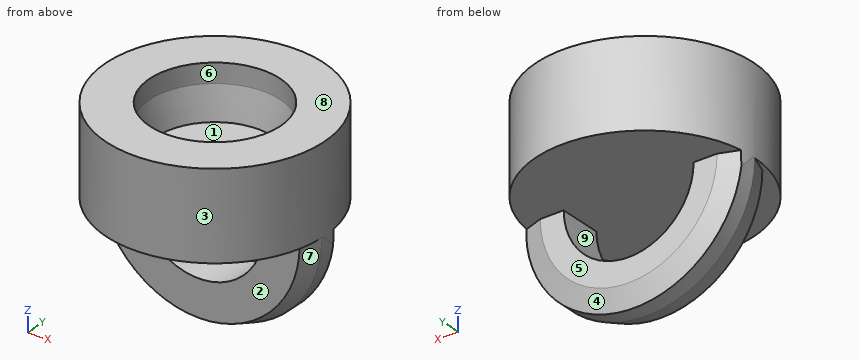
from build123d import *

# Parameters (mm, degrees)
SKETCH1_R                = 7.5
BOSS_EXTRUDE1_DEPTH      = 6
SKETCH2_R                = 4.5
CUT_EXTRUDE1_DEPTH       = 3.5
CHAMFER1_SIZE            = 0.5
CHAMFER1_SIZE2           = 2.165737937
BOSS_EXTRUDE2_DEPTH      = 1.5
BOSS_EXTRUDE2_DEPTH_BACK = 1.5
SKETCH4_OUTSIDE_W        = 22.028
SKETCH4_OUTSIDE_H        = 22.028
SKETCH4_OUTSIDE_R        = 7.5
CUT_EXTRUDE2_DEPTH       = 13.990381057
CHAMFER3_SIZE            = 1.37373871
CHAMFER3_SIZE_2          = 0.5


with BuildPart() as part:
    # Sketch1 → Boss-Extrude1 (new body)
    with BuildSketch(Plane.XY):
        Circle(SKETCH1_R)
    extrude(amount=BOSS_EXTRUDE1_DEPTH)

    # Sketch2 → Cut-Extrude1 (cut)
    with BuildSketch(Plane.XY.offset(6)):
        Circle(SKETCH2_R)
    extrude(amount=-CUT_EXTRUDE1_DEPTH, mode=Mode.SUBTRACT)

    # Chamfer1
    chamfer1_edges = [part.edges().sort_by_distance(p)[0] for p in [
        (-4.5, 0, 2.5),
    ]]
    chamfer1_side = [part.faces().sort_by_distance(p)[0] for p in [
        (0, 0, 2.5),
    ]]
    chamfer(chamfer1_edges, length=CHAMFER1_SIZE, length2=CHAMFER1_SIZE2, reference=chamfer1_side[0])

    # Sketch3 → Boss-Extrude2 (add, two sides: drawn at the far end of the back side and taken through both)
    with BuildSketch(Plane(origin=(0, 0, 0), x_dir=(1, 0, 0), z_dir=(0, 1, 0)).offset(-BOSS_EXTRUDE2_DEPTH_BACK)):
        with BuildLine():
            Line((-7.5, 0), (-4.5, 0))
            ThreePointArc((-4.5, 0), (0, 4.5), (4.5, 0))
            Line((4.5, 0), (7.5, 0))
            ThreePointArc((7.5, 0), (0, 7.5), (-7.5, 0))
        make_face()
    extrude(amount=BOSS_EXTRUDE2_DEPTH + BOSS_EXTRUDE2_DEPTH_BACK)

    # Sketch4 outside → Cut-Extrude2 (cut, through all)
    with BuildSketch(Plane.XY):
        Rectangle(SKETCH4_OUTSIDE_W, SKETCH4_OUTSIDE_H)
        Circle(SKETCH4_OUTSIDE_R, mode=Mode.SUBTRACT)
    extrude(amount=-CUT_EXTRUDE2_DEPTH, mode=Mode.SUBTRACT)

    # Chamfer3
    # the kernel refuses this chamfer: 1.37373871, 0.5 mm, written as the material it takes off along each edge
    with BuildSketch(Plane(origin=(0, -1.5, 0), x_dir=(0.9625909817516988, 0, 0.27095867184923395), z_dir=(-0.27095867184923395, 0, 0.9625909817516988))) as chamfer3_piece_1_section:
        Polygon((7.5, CHAMFER3_SIZE), (7.5 - CHAMFER3_SIZE_2, 0), (7.5, 0), align=None)
    chamfer3_piece_1 = revolve(axis=Axis((0, -1.5, 0), (0, 1, 0)), revolution_arc=211.442642735, mode=Mode.PRIVATE)
    chamfer3_piece_1 = split(chamfer3_piece_1, bisect_by=Plane(origin=(0, -0.82033622, 0), z_dir=(0, 0, -1)), keep=Keep.TOP, mode=Mode.PRIVATE)
    add(chamfer3_piece_1, mode=Mode.SUBTRACT)
    with BuildSketch(Plane(origin=(0, 1.5, 0), x_dir=(0.9625909817516987, 0, 0.2709586718492343), z_dir=(-0.2709586718492343, 0, 0.9625909817516987))) as chamfer3_piece_2_section:
        Polygon((7.5 - CHAMFER3_SIZE, 0), (7.5, -CHAMFER3_SIZE_2), (7.5, 0), align=None)
    chamfer3_piece_2 = revolve(axis=Axis((0, 1.5, 0), (0, 1, 0)), revolution_arc=211.442642735, mode=Mode.PRIVATE)
    chamfer3_piece_2 = split(chamfer3_piece_2, bisect_by=Plane(origin=(0, 1.269508832, 0), z_dir=(0, 0, -1)), keep=Keep.TOP, mode=Mode.PRIVATE)
    add(chamfer3_piece_2, mode=Mode.SUBTRACT)


solid = part.part
Source: CAD feature listing. Evaluate the final solid. Frame: model axes, mm. Face numbers are marked on the shaded views. A direction names the side the tool comes from. Give positions to 0.01 mm unless a question says otherwise; leave off trailing zeros. Write each loop counter-clockwise with the first axis right and the second up, starting at its lowest first coordinate (ties: lowest second). Pieces come first, ordered by that corner, then holes. Notation, with made-up numbers: M 85.5,70 L 94.5,70 A24 ccw 94.5,101 Z; hole C 48.25,66 d4. An arc over 180 degrees is marked long. Return JSON: item names as keys, results as strings. Group by question number.
1) Pull-direction query (Y, two-part tool) for the marked faces 1, 2, 3 and 4; classes: pulls with the +Y half, pulls with the -Y half, needs draft (parallel to the pull), parting line crosses it, or undercut.
2) Cut plane A-A, the plane x = 0. Output: boundary loops of the cut face in (y, z).
3) Cut plane D-D, the plane y = -6.25. Output: boundary loops of the cut face in (x, z).
4) Set-up query: the marked faces 5, 6, 7, 8 and 9. Return all of +Z, -Z, +X, -X, +Y, -Y with unobstructed straight access to the full face (end or side cutting, diameter ignored); none if empty.
5) Material intervals for line 1 along Y through (x, z) = (0, 5.1); line 2 along Z through (x, y) = (-1, 6); line 3 along Z through (x, y) = (0.25, 2.75), sorted ascending. Write a range as [from, to].
6) Cut plane C-C, the plane y = 5.5. Output: boundary loops of the cut face in (x, z).
7) Cut plane B-B, the plane z = 1.5. Output: boundary loops of the cut face in (x, y), plus the area to 3 significant figures.
8) Pin query (flat end, axial travel): P1, Ø5, axis at y = 5, z = -1.5, coming from the -X side; P2, Ø5, axis at x = 2.5, z = -4, coming from the +Y side; P3, Ø4, axis at x = 0, y = -0.5, coming from the +Z side. Return the tip coordinate at first contact, or that it passes through.
Recorded:
{
 "1": {"face 1": "undercut", "face 2": "pulls with the -Y half", "face 3": "parting line crosses it", "face 4": "pulls with the +Y half"},
 "2": {"outline": "M -7.5,0 L 7.5,0 L 7.5,6 L 4.5,6 L 4.5,4.67 L 4,2.5 L -4,2.5 L -4.5,4.67 L -4.5,6 L -7.5,6 Z; M -1.5,-7 L -0.13,-7.5 L 1,-7.5 L 1.5,-6.13 L 1.5,-4.5 L -1.5,-4.5 Z"},
 "3": {"outline": "M -4.15,0 L 4.15,0 L 4.15,6 L -4.15,6 Z"},
 "4": {"face 5": "-Z, +X, -X, +Y", "face 6": "+Z", "face 7": "-Z, -Y", "face 8": "+Z, +X, -X, +Y, -Y", "face 9": "+Y, -Y"},
 "5": {"line 1": "y = [-7.5, -4.5], [4.5, 7.5]", "line 2": "z = [0, 6]", "line 3": "z = [0, 2.5]"},
 "6": {"outline": "M -5.1,0 L 5.1,0 L 5.1,6 L -5.1,6 Z"},
 "7": {"outline": "C 0,0 d15", "area": "177 mm²"},
 "8": {"P1": "stops at x = -6.87", "P2": "stops at y = 1.5", "P3": "stops at z = 2.5"}
}
